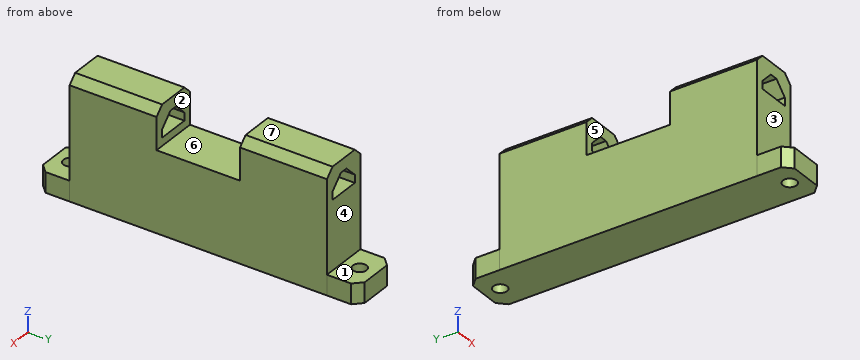
from build123d import *

# Parameters (mm, degrees)
F0_W     = 12.022123
F0_H     = 8
F0_R     = 1.7
F1_DEPTH = 5
F2_DEPTH = 30
F3_DEPTH = 20
F4_W     = 8
F4_H     = 5
F5_DEPTH = 72.001
F6_SIZE  = 3
F7_SIZE  = 2


with BuildPart() as f1:
    # F0 (on Top) → F1 (new body)
    with BuildSketch(Plane.XY):
        with Locations((35.656364, -18.254959)):
            Rectangle(F0_W, F0_H)
        with Locations((35.656365, -18.254959)):
            Circle(F0_R, mode=Mode.SUBTRACT)
        Polygon((41.667426, -22.254959), (29.645303, -22.254959), (29.645303, -43.874378), (35.656365, -43.874378), (41.667426, -43.874378), align=None)
        Polygon((35.656365, -43.874378), (29.645303, -43.874378), (29.645303, -54.254959), (29.645303, -64.63554), (35.656365, -64.63554), (41.667426, -64.63554), (41.667426, -54.254959), (41.667426, -43.874378), align=None)
        Polygon((35.656365, -64.63554), (29.645303, -64.63554), (29.645303, -86.254959), (41.667426, -86.254959), (41.667426, -64.63554), align=None)
        with Locations((35.656364, -90.254959)):
            Rectangle(F0_W, F0_H)
        with Locations((35.656365, -90.254959)):
            Circle(F0_R, mode=Mode.SUBTRACT)
    extrude(amount=F1_DEPTH)

    # F0 (on Top) → F2 (join)
    with BuildSketch(Plane.XY):
        Polygon((41.667426, -22.254959), (29.645303, -22.254959), (29.645303, -43.874378), (35.656365, -43.874378), (41.667426, -43.874378), align=None)
        Polygon((35.656365, -64.63554), (29.645303, -64.63554), (29.645303, -86.254959), (41.667426, -86.254959), (41.667426, -64.63554), align=None)
    extrude(amount=F2_DEPTH)

    # F0 (on Top) → F3 (join)
    with BuildSketch(Plane.XY):
        Polygon((35.656365, -43.874378), (29.645303, -43.874378), (29.645303, -54.254959), (29.645303, -64.63554), (35.656365, -64.63554), (41.667426, -64.63554), (41.667426, -54.254959), (41.667426, -43.874378), align=None)
    extrude(amount=F3_DEPTH)

    # F4 (on face) → F5 (cut, through all)
    with BuildSketch(Plane.XZ.offset(86.254959)):
        with Locations((35.656365, 24.5)):
            Rectangle(F4_W, F4_H)
    extrude(amount=-F5_DEPTH, mode=Mode.SUBTRACT)

    # F6
    f6_edges = [f1.edges().sort_by_distance(p)[0] for p in [
        (31.656365, -75.44525, 27),
        (31.656365, -33.064669, 27),
        (39.656365, -75.44525, 27),
        (39.656365, -33.064669, 27),
    ]]
    chamfer(f6_edges, length=F6_SIZE)

    # F7
    f7_edges = [f1.edges().sort_by_distance(p)[0] for p in [
        (29.645303, -94.254959, 2.5),
        (41.667426, -94.254959, 2.5),
        (29.645303, -14.254959, 2.5),
        (41.667426, -14.254959, 2.5),
        (41.667426, -33.064669, 30),
        (29.645303, -33.064669, 30),
        (29.645303, -75.44525, 30),
        (41.667426, -75.44525, 30),
    ]]
    chamfer(f7_edges, length=F7_SIZE)


solid = f1.part
Verification items for the finished model (mm, model axes). Face numbers are marked on the shaded views. A direction names the side the tool comes from. Give positions to 0.01 mm unless a question says otherwise; leave off trailing zeros. Write each loop counter-clockwise with the first axis right and the second up, starting at its lowest first coordinate (ties: lowest second). Pieces come first, ordered by that corner, then holes. Notation, with made-up numbers: M 85.25,81.5 L 144.25,81.5 A14 cw 144.25,89.5 Z; hole C 72,-33 d9. An arc over 180 degrees is marked long. Use CSV: the item, a comma, the result in double quotes.
1) Cross-section at B-B (y = -38). Enter the section's corners in (x, z), plus the area to 3 significant figures.
Final values:
outline,"M 29.65,0 L 41.67,0 L 41.67,28 L 39.67,30 L 31.65,30 L 29.65,28 Z; hole M 31.66,22 L 39.66,22 L 39.66,24 L 36.66,27 L 34.66,27 L 31.66,24 Z"
area,"326 mm²"
2) Release check for a two-part mould opening along Y. For the marked faces 4, 5, 6 and 7 record: released by +Y, released by -Y, zero draft, split by the parting line, or undercut.
Final values:
face 4,"released by +Y"
face 5,"undercut"
face 6,"undercut"
face 7,"zero draft"
3) Cross-section at C-C (z = 3.5). Enter the section's corners in (x, y), plus the area to 3 significant figures.
Final values:
outline,"M 29.65,-92.25 L 31.65,-94.25 L 39.67,-94.25 L 41.67,-92.25 L 41.67,-16.25 L 39.67,-14.25 L 31.65,-14.25 L 29.65,-16.25 Z; hole C 35.66,-90.25 d3.4; hole C 35.66,-18.25 d3.4"
area,"936 mm²"
4) Go/stop test with flat-tipped pins: pin 1 Ø5 at (x, z) = (38, 24) entering from +Y; pin 2 Ø2 at (x, y) = (35.66, -18.25) entering from +Z; pin 3 Ø4 at (x, y) = (35.66, -90.25) entering from +Z; pin 4 Ø5 at (x, z) = (34, 23) entering from -Y. Record where each tip stops, or that it passes through.
Final values:
pin 1,"y = -22.25"
pin 2,"through"
pin 3,"z = 5"
pin 4,"y = -86.25"
5) Cross-section at D-D (y = -46.5). Enter the section's corners in (x, z).
Final values:
outline,"M 29.65,0 L 41.67,0 L 41.67,20 L 29.65,20 Z"
6) Material ranges on line 1 along Y through (x, z) = (32, 27); line 2 along Z through (x, y) = (34.75, -76.5); line 3 along Y through (x, z) = (30, 13), recorded low to high.
Final values:
line 1,"-86.25 to -64.64, -43.87 to -22.25"
line 2,"0 to 22, 27 to 30"
line 3,"-86.25 to -22.25"
7) Cross-section at A-A (z = 23). Enter the section's corners in (x, y).
Final values:
outline,"M 29.65,-86.25 L 31.66,-86.25 L 31.66,-64.64 L 29.65,-64.64 Z; M 29.65,-43.87 L 31.66,-43.87 L 31.66,-22.25 L 29.65,-22.25 Z; M 39.66,-86.25 L 41.67,-86.25 L 41.67,-64.64 L 39.66,-64.64 Z; M 39.66,-43.87 L 41.67,-43.87 L 41.67,-22.25 L 39.66,-22.25 Z"
8) Access from +Z, -Z, +X, -X, +Y, -Y to the whole of each face (thin tool, end or side, straight path). Record for the marked faces 1, 2 and 3.
Final values:
face 1,"+Z, +X, -X, +Y"
face 2,"+Z, +X, -X"
face 3,"+Z, +X, -X, -Y"
